Answer from the drawing. Dimensions are ordinates in mm from the lowest x, y and z of the part. Coordinates: 2 decimals unless noted, no trailing zeros. Order: outer loops, then holes, each group sorted by start corner. A loop starts at its lowest first (then second) coordinate and runs counter-clockwise, first axis right, second up. Notation, with made-up numbers: (-2.75, 29.5) -> (39.25, 29.5) arc R4 cw to (39.25, 34.5) -> close; hole circle Ø9 at (-30.75, 7.25). An arc over 180 degrees is marked (long way). Answer in a Markdown table with one row per item.
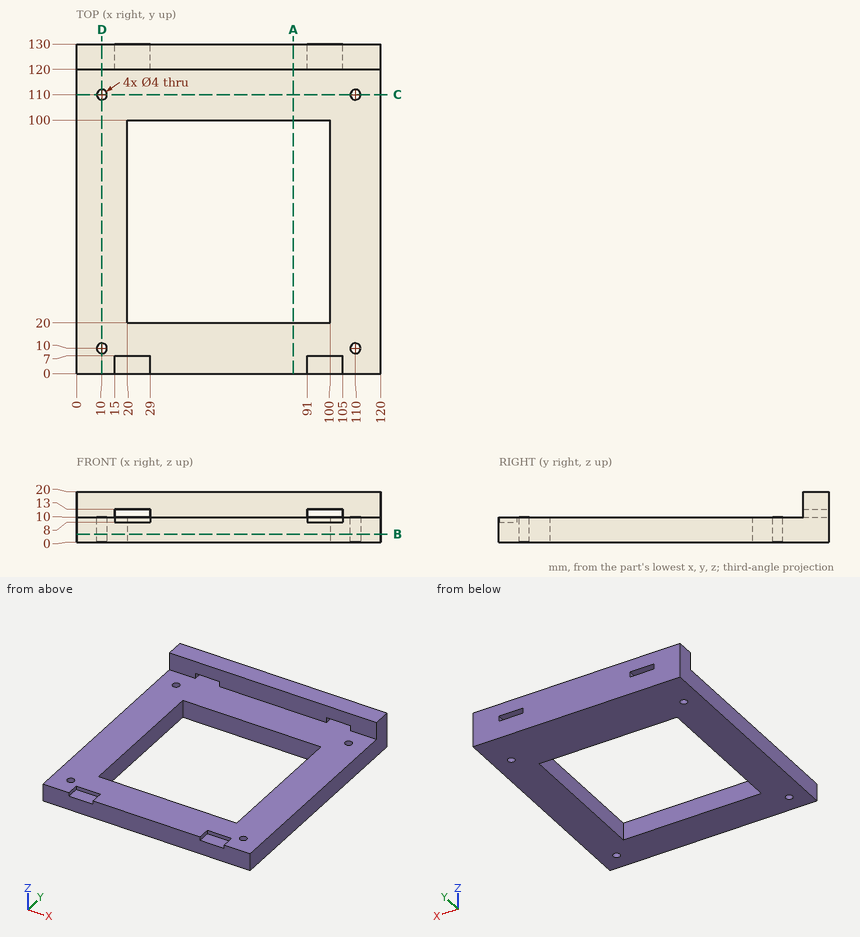
Q1. Consider line 1 (Y direction, x = 110, z = 6.25); line 2 (X direction, y = 110, z = 3.75); line 3 (X direction, y = 56, z = 7.75). Determine where each line is inside the solid, lowest interval first.
Outcome:
| item | result |
|---|---|
| line 1 | 0 to 8, 12 to 108, 112 to 130 |
| line 2 | 0 to 8, 12 to 108, 112 to 120 |
| line 3 | 0 to 20, 100 to 120 |
Q2. The part is cut by section C-C (y = 110). Write down the section's boundary in (x, z), then the cut area to 3 significant figures.
Outcome:
| item | result |
|---|---|
| outline | (0, 0) -> (8, 0) -> (8, 10) -> (0, 10) -> close; (12, 0) -> (108, 0) -> (108, 10) -> (12, 10) -> close; (112, 0) -> (120, 0) -> (120, 10) -> (112, 10) -> close |
| area | 1,120 mm² |
Q3. The part is cut by section D-D (x = 10). Write down the section's boundary in (y, z).
Outcome:
| item | result |
|---|---|
| outline | (0, 0) -> (8, 0) -> (8, 10) -> (0, 10) -> close; (12, 0) -> (108, 0) -> (108, 10) -> (12, 10) -> close; (112, 0) -> (130, 0) -> (130, 20) -> (120, 20) -> (120, 10) -> (112, 10) -> close |
Q4. The part is cut by section B-B (z = 3.25). Write down the section's boundary in (x, y), then the cut area to 3 significant figures.
Outcome:
| item | result |
|---|---|
| outline | (0, 0) -> (120, 0) -> (120, 130) -> (0, 130) -> close; hole circle Ø4 at (10, 10); hole circle Ø4 at (10, 110); hole (20, 20) -> (100, 20) -> (100, 100) -> (20, 100) -> close; hole circle Ø4 at (110, 10); hole circle Ø4 at (110, 110) |
| area | 9,150 mm² |
Q5. The part is cut by section A-A (x = 85.5). Write down the section's boundary in (y, z), then the cut area to 3 significant figures.
Outcome:
| item | result |
|---|---|
| outline | (0, 0) -> (20, 0) -> (20, 10) -> (0, 10) -> close; (100, 0) -> (130, 0) -> (130, 20) -> (120, 20) -> (120, 10) -> (100, 10) -> close |
| area | 600 mm² |
Q6. Given pin 1 (4.5 mm diameter, centred on x = 10, y = 110, fed in from +Z); pin 2 (5.5 mm diameter, centred on x = 21.5, y = 4, fed in from +Z); pin 3 (3 mm diameter, centred on x = 62.5, z = 17, fed in from -Y), each flat-ended and moving along its own axis, determine where each tip first touches the part or whether it passes through.
Outcome:
| item | result |
|---|---|
| pin 1 | z = 10 |
| pin 2 | z = 8 |
| pin 3 | y = 120 |
